Source: CAD feature listing. Evaluate the final solid. Frame: model axes, mm. Face numbers are marked on the shaded views. A direction names the side the tool comes from. Round coordinates to 2 decimals unless told otherwise and drop trailing zeros. Order: outer loops, then holes, each group sorted by start corner. A loop starts at its lowest first (then second) coordinate and runs counter-clockwise, first axis right, second up. Notation, with made-up numbers: M 16.5,30.5 L 55.5,30.5 A24 ccw 55.5,56.5 Z; hole C -25.5,48 d11. An arc over 180 degrees is marked long. Use one line per item in the form item = value. Start each with the question number.
Q1. Section D-D (z = 40.5). Return the cut outline in (x, y), plus the area to 3 significant figures.
Q2. Section C-C (z = 3.5). Return the cut outline in (x, y), plus the area to 3 significant figures.
Q3. Material intervals for probe 1 along Z at (x, y) = (-9.5, 4.75); probe 2 along Z at (x, y) = (-1.5, 1.5); probe 3 along X at (y, z) = (-0.25, 17.5), sorted ascending.
Q4. Section A-A (z = 15). Return the cut outline in (x, y).
Q5. Pull-direction query (X, two-part tool) for the marked faces 3, 4 and 5; classes: pulls with the +X half, pulls with the -X half, needs draft (parallel to the pull), parting line crosses it, or undercut.
Q6. Contact query for flat-ended pins moving along their axis: pin 1 (10 mm diameter, centred on x = -3, y = 8, fed in from +Z); pin 2 (12 mm diameter, centred on y = 0.5, z = 18, fed in from +X); pin 3 (2 mm diameter, centred on y = 3.5, z = 3.5, fed in from -X). Output: stop coordinate, or through.
Q7. Reachability of the marked faces 1 and 2 from +Z, -Z, +X, -X, +Y, -Y: full face, straight path, thin tool, end or side. Return the list, or none.
Q8. Section B-B (y = 6.75). Return the cut outline in (x, z), plus the area to 3 significant figures.
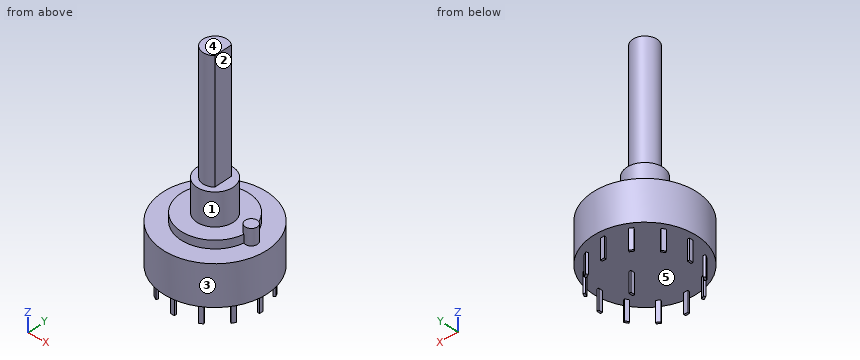
from build123d import *

# Parameters (mm, degrees)
CYLINDER001_R     = 8.5
CYLINDER001_DEPTH = 2
BOX_W             = 0.5
BOX_H             = 1
BOX_DEPTH         = 5
ARRAY_COUNT       = 12
BOX001_W          = 0.5
BOX001_H          = 1
BOX001_DEPTH      = 5
CYLINDER002_R     = 4.5
CYLINDER002_DEPTH = 8
CYLINDER004_R     = 1.5
CYLINDER004_DEPTH = 4
BOX002_W          = 1
BOX002_H          = 10
BOX002_DEPTH      = 30
CYLINDER003_R     = 3
CYLINDER003_DEPTH = 30
CYLINDER_R        = 13
CYLINDER_DEPTH    = 10


with BuildPart() as cylinder001:
    # Cylinder001 → Cylinder001 (new body)
    with BuildSketch(Plane.XY.offset(10)):
        Circle(CYLINDER001_R)
    extrude(amount=CYLINDER001_DEPTH)


with BuildPart() as pin_array:
    # Box → Box (new body)
    with BuildSketch(Plane(origin=(11, -0.5, -5), x_dir=(1, 0, 0), z_dir=(0, 0, 1))):
        with Locations((0.25, 0.5)):
            Rectangle(BOX_W, BOX_H)
    extrude(amount=BOX_DEPTH)

    # Array: Pin array ×12 about axis
    array_axis = Axis((0, 0, 0), (0, 0, 1))


with BuildPart() as pin_array_1:
    add(pin_array.part)
    for i in range(1, ARRAY_COUNT):
        add(pin_array.part.rotate(array_axis, i * 360 / ARRAY_COUNT))


with BuildPart() as pin_central:
    # Box001 → Box001 (new body)
    with BuildSketch(Plane(origin=(3, -0.5, -5), x_dir=(1, 0, 0), z_dir=(0, 0, 1))):
        with Locations((0.25, 0.5)):
            Rectangle(BOX001_W, BOX001_H)
    extrude(amount=BOX001_DEPTH)


with BuildPart() as cylinder002:
    # Cylinder002 → Cylinder002 (new body)
    with BuildSketch(Plane.XY.offset(12)):
        Circle(CYLINDER002_R)
    extrude(amount=CYLINDER002_DEPTH)


with BuildPart() as cylinder004:
    # Cylinder004 → Cylinder004 (new body)
    with BuildSketch(Plane(origin=(9, 0, 10), x_dir=(1, 0, 0), z_dir=(0, 0, 1))):
        Circle(CYLINDER004_R)
    extrude(amount=CYLINDER004_DEPTH)


with BuildPart() as obj1:
    # Box002 → Box002 (new body)
    with BuildSketch(Plane(origin=(2, -5, 20), x_dir=(1, 0, 0), z_dir=(0, 0, 1))):
        with Locations((0.5, 5)):
            Rectangle(BOX002_W, BOX002_H)
    extrude(amount=BOX002_DEPTH)


with BuildPart() as obj2:
    # Cylinder003 → Cylinder003 (new body)
    with BuildSketch(Plane.XY.offset(20)):
        Circle(CYLINDER003_R)
    extrude(amount=CYLINDER003_DEPTH)

    # Cut: cut obj1
    add(obj1.part, mode=Mode.SUBTRACT)


with BuildPart() as selector_final:
    # Cylinder → Cylinder (new body)
    with BuildSketch(Plane.XY):
        Circle(CYLINDER_R)
    extrude(amount=CYLINDER_DEPTH)

    # Fusion: union Cylinder001, Pin array, Pin central, Cylinder002, Cylinder004, obj2
    add(cylinder001.part)
    add(pin_array_1.part)
    add(pin_central.part)
    add(cylinder002.part)
    add(cylinder004.part)
    add(obj2.part)


solid = selector_final.part
Results list:
q1.outline = M 2,-2.24 L 2,2.24 A3 ccw long Z
q1.area = 25.2 mm2
q2.outline = C 0,0 d26
q2.area = 531 mm2
q3.probe_1 = 0 to 10
q3.probe_2 = 0 to 50
q3.probe_3 = -4.49 to 4.49
q4.outline = C 0,0 d9
q5.face_3 = parting line crosses it
q5.face_4 = needs draft
q5.face_5 = undercut
q6.pin_1 = 20
q6.pin_2 = 10.5
q6.pin_3 = -12.76
q7.face_1 = +Z
q7.face_2 = +Z, +X, +Y, -Y
q8.outline = M -11.11,0 L 11.11,0 L 11.11,10 L 5.17,10 L 5.17,12 L -5.17,12 L -5.17,10 L -11.11,10 Z
q8.area = 243 mm2
